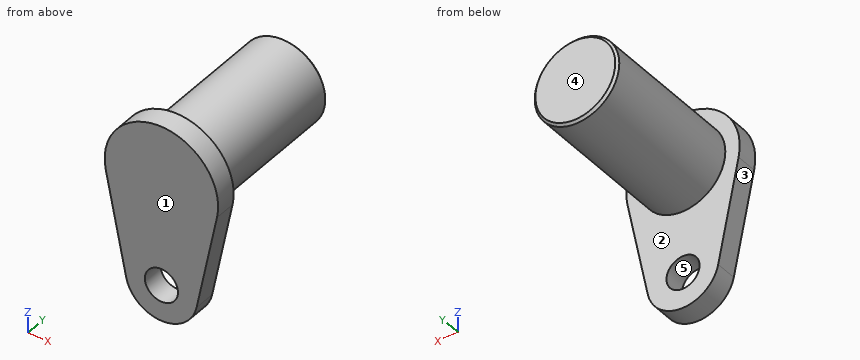
from build123d import *

# Parameters (mm, degrees)
F0_R     = 3.5
F1_DEPTH = 4.6
F2_R     = 8.95
F3_DEPTH = 31.8
F4_SIZE  = 0.5


with BuildPart() as f1:
    # F0 (on Front) → F1 (new body)
    with BuildSketch(Plane.XZ):
        with BuildLine():
            Line((7.446449, -23.52), (11.757551, -2.4))
            ThreePointArc((11.757551, -2.4), (0, 12), (-11.757551, -2.4))
            Line((-11.757551, -2.4), (-7.446449, -23.52))
            ThreePointArc((-7.446449, -23.52), (0, -29.6), (7.446449, -23.52))
        make_face()
        with Locations((0, -22)):
            Circle(F0_R, mode=Mode.SUBTRACT)
    extrude(amount=F1_DEPTH)

    # F2 (on face) → F3 (join)
    with BuildSketch(Plane(origin=(0, 0, 0), x_dir=(-1, 0, 0), z_dir=(0, 1, 0))):
        Circle(F2_R)
    extrude(amount=F3_DEPTH)

    # F4
    f4_edges = [f1.edges().sort_by_distance(p)[0] for p in [
        (8.95, 31.8, 0),
    ]]
    chamfer(f4_edges, length=F4_SIZE)


solid = f1.part
Geometry check sheet. Reference: the model listing, model coordinates, mm. Face numbers are marked on the shaded views. A direction names the side the tool comes from. Give positions to 0.01 mm unless a question says otherwise; leave off trailing zeros. Order: outer loops, then holes, each group sorted by start corner. A loop starts at its lowest first (then second) coordinate and runs counter-clockwise, first axis right, second up.
1) Cross-section at A-A (x = 0). Record the boundary of the cut face in (y, z).
Results are:
outline: (-4.6, -29.6) - (0, -29.6) - (0, -25.5) - (-4.6, -25.5) - close; (-4.6, -18.5) - (0, -18.5) - (0, -8.95) - (31.3, -8.95) - (31.8, -8.45) - (31.8, 8.45) - (31.3, 8.95) - (0, 8.95) - (0, 12) - (-4.6, 12) - close
2) Cross-section at D-D (z = 0). Record the boundary of the cut face in (x, y).
Results are:
outline: (-12, -4.6) - (12, -4.6) - (12, 0) - (8.95, 0) - (8.95, 31.3) - (8.45, 31.8) - (-8.45, 31.8) - (-8.95, 31.3) - (-8.95, 0) - (-12, 0) - close
3) Draft check along X on the marked faces 3, 4 and 5. Enter one of: released by +X, released by -X, zero draft, split by the parting line, or undercut.
Results are:
face 3: released by -X
face 4: zero draft
face 5: undercut
4) Material ranges on probe 1 along Y at (x, z) = (7.75, -16); probe 2 along X at (y, z) = (1.5, 8); probe 3 along Z at (x, y) = (5.25, 17), recorded low to high.
Results are:
probe 1: y = -4.6 to 0
probe 2: x = -4.01 to 4.01
probe 3: z = -7.25 to 7.25
5) Gauge pin test, flat ends, axial feed: pin 1 (1.5 mm diameter, centred on x = 5.5, y = 14, fed in from +Z); pin 2 (3 mm diameter, centred on x = -5.5, y = 7.5, fed in from +Z); pin 3 (3 mm diameter, centred on y = 1, z = -16.5, fed in from +X). Record the tip position at first contact, or that the pin passes through.
Results are:
pin 1: stops at z = 7.59
pin 2: stops at z = 8.01
pin 3: stops at x = 9.11
6) Cross-section at B-B (z = -22). Record the boundary of the cut face in (x, y).
Results are:
outline: (-7.76, -4.6) - (-3.5, -4.6) - (-3.5, 0) - (-7.76, 0) - close; (3.5, -4.6) - (7.76, -4.6) - (7.76, 0) - (3.5, 0) - close
7) Cross-section at C-C (y = -1.5). Record the boundary of the cut face in (x, z).
Results are:
outline: (-11.76, -2.4) - (-7.45, -23.52) arc R7.6 ccw to (7.45, -23.52) - (11.76, -2.4) arc R12 ccw (long way) to start; hole circle Ø7 at (0, -22)
8) Tool access check on the marked faces 1 and 2. Record the directions out of +Z, -Z, +X, -X, +Y, -Y that give a thin tool (end or side, any length) a straight path to the whole face; none if there is none.
Results are:
face 1: +Z, -Z, +X, -X, -Y
face 2: +Y
